Autodesk Inventor part; units mm, degrees
ref_plane "YZ Plane" through (0, 0, 0) normal (1, 0, 0) x (0, 1, 0)
ref_plane "XZ Plane" through (0, 0, 0) normal (0, 1, 0) x (-1, 0, 0)
ref_plane "XY Plane" through (0, 0, 0) normal (0, 0, 1) x (1, 0, 0)
sketch "Sketch1" plane through (0, 0, 0) normal (0, 0, 1) x (1, 0, 0)
  circle A0 centre (0, 0) radius 229
  circle A1 centre (0, 0) radius 301
  circle A2 centre (0, 0) radius 265 construction
  line L0 (0, 229) -> (0, 301) construction
  point P0 (0, 265)
  dimension "d17" = 530
  dimension "d18" = 72
extrude "Extrusion1" add sketch "Sketch1" along normal blind 15
sketch "Sketch2" plane through (0, 0, 15) normal (0, 0, 1) x (1, 0, 0)
  circle A0 centre (0, 0) radius 301 construction
  circle A1 centre (0, 0) radius 229 construction
  line L0 (0, 286) -> (0, 244) construction
  line L1 (0, 229) -> (0, 0) construction
  circle A2 centre (0, 0) radius 244
  circle A3 centre (0, 0) radius 286
  circle A4 centre (0, 0) radius 265 construction
  point P0 (0, 265)
  dimension "d19" = 530
  dimension "d4" = 42
extrude "Extrusion2" cut sketch "Sketch2" against normal blind 3.5
sketch "Sketch3" plane through (0, 0, 0) normal (0, 0, 1) x (1, 0, 0)
  circle A0 centre (0, 0) radius 229 construction
  circle A1 centre (0, 0) radius 301 construction
  circle A2 centre (0, 0) radius 244
  circle A3 centre (0, 0) radius 286
  circle A4 centre (0, 0) radius 301
  line L0 (0, 0) -> (0, -301) construction
  line L1 (0, 0) -> (58.7222, -295.2164) construction
  line L2 (47.602, -239.3116) -> (55.7958, -280.5046) construction
  circle A5 centre (51.6989, -259.9081) radius 7
  dimension "d20" = 11.25
  dimension "d21" = 14
extrude "Extrusion3" cut sketch "Sketch3" along normal through all contours A5
pattern_circular "Circular Pattern2" count 8 over 157.5 about axis through (0, 0, 0) along (0, 0, -1) of "Extrusion3" both ways yes
sketch "Sketch5" plane through (0, 0, 0) normal (0, 0, -1) x (-1, 0, 0)
  circle A0 centre (0, 0) radius 301
  circle A1 centre (0, 0) radius 229
  line L0 (0, 0) -> (0, 229) construction
  arc A2 (2.5, 228.9864) -> (-2.5, 228.9864) centre (0, 229) ccw
  dimension "d40" = 5
extrude "Extrusion4" cut sketch "Sketch5" against normal through all contours A1 A2
mirror "Mirror1" about plane through (0, 0, 0) normal (0, 1, 0) of "Extrusion4"
equation "\"d17\" = Шпил_пласт_КОРМА_диам_центров"
equation "\"d19\" = Шпил_пласт_КОРМА_диам_центров"
equation "\"BendReliefDepth\" = 0.5 * Thickness"
properties part number "ДМФ 022 кольцо прижимное корма внутреннее"
Model file for the job. Use its own axes, mm. A direction names the side the tool comes from. Round coordinates to 2 decimals unless told otherwise and drop trailing zeros. Order: outer loops, then holes, each group sorted by start corner. A loop starts at its lowest first (then second) coordinate and runs counter-clockwise, first axis right, second up.
(1) 3-axis set-ups, long thin cutter, end or side, ignore diameter. For faces 1 (the face through (266, -110, 15)), 2 (the face through (-228.945, -5.001, 7.395)), 3 (the face through (-210.794, 193.292, 13.274)): which of +Z, -Z, +X, -X, +Y, -Y reach the whole face in a straight line?
(2) Band-saw the part on C-C (z = 8.25). Give the number of separate pieces and of enclosed holes in the cut face, then the cut area to 3 significant figures.
(3) Pin check, flat tips, straight feed: pin 1 (12.5 mm diameter, centred on x = 220.34, y = -147.23, fed in from +Z); pin 2 (1.5 mm diameter, centred on y = 159.5, z = 3, fed in from +X); pin 3 (16 mm diameter, centred on x = -259.91, y = -51.7, fed in from +Z); pin 4 (5 mm diameter, centred on x = 51.5, z = 12, fed in from -Y). Stop position of each tip, or through.
(4) Pull direction Y, two halves, no side cores. Call faces 4 (the face through (228.945, 5.001, 7.395)), 5 (the face through (-221.85, -203.43, 7.4)), 6 (the face through (65, 224, 0)): released by +Y, released by -Y, zero draft, split by the parting line, or undercut.
(5) Drill centre lines: line 1 (Y direction, x = 0, z = 12.5); line 2 (Y direction, x = -194.5, z = 13.5); line 3 (X direction, y = -259, z = 10.75). Where is each one in solid material? Low to high.
(6) Band-saw the part on B-B (x = -36). List the corners of the cut face in (y, z).
(7) Band-saw the part on A-A (y = 0). List the corners of the cut face in (x, z), then the cut area to 3 significant figures.
Verdict:
1. face 1: +Z, +X, -X, +Y, -Y
1. face 2: +Z, -Z
1. face 3: +Z
2. separate pieces: 1
2. enclosed holes: 9
2. area: 119,000 mm2
3. pin 1: passes through
3. pin 2: stops at x = 255.73
3. pin 3: stops at z = 11.5
3. pin 4: stops at y = -296.98
4. face 4: undercut
4. face 5: split by the parting line
4. face 6: zero draft
5. line 1: y = -301 to -286, -244 to -231.5, 231.5 to 244, 286 to 301
5. line 2: y = -229.72 to -209.68, -147.33 to -120.87, 120.87 to 147.33, 209.68 to 229.72
5. line 3: x = -153.36 to -58.64, -44.76 to 44.76, 58.64 to 153.36
6. outline: (-298.84, 0) - (-226.15, 0) - (-226.15, 15) - (-241.33, 15) - (-241.33, 11.5) - (-283.73, 11.5) - (-283.73, 15) - (-298.84, 15) - close; (226.15, 0) - (298.84, 0) - (298.84, 15) - (283.73, 15) - (283.73, 11.5) - (241.33, 11.5) - (241.33, 15) - (226.15, 15) - close
7. outline: (-301, 0) - (-229, 0) - (-229, 15) - (-244, 15) - (-244, 11.5) - (-286, 11.5) - (-286, 15) - (-301, 15) - close; (229, 0) - (301, 0) - (301, 15) - (286, 15) - (286, 11.5) - (244, 11.5) - (244, 15) - (229, 15) - close
7. area: 1,870 mm2
